Verification items for this drawing (mm, ordinates from the low corner). Round coordinates to 2 decimals unless told otherwise and drop trailing zeros. Loops run counter-clockwise (first coordinate to the right, second up) from the corner with the lowest first, then second, coordinate; pieces in that order, holes last. Notation, with made-up numbers: (14.5, 68.25) - (34.5, 68.25) arc R8 cw to (34.5, 81.25) - close; hole circle Ø4 at (38.5, 38.5). An arc over 180 degrees is marked (long way). Answer in a Markdown table with one row per item. Add a question column.
(1) Gauge pin test, flat ends, axial feed: pin 1 (3 mm diameter, centred on x = 25.5, z = 126, fed in from -Y); pin 2 (4 mm diameter, centred on x = 37.5, z = 14, fed in from -Y); pin 3 (3 mm diameter, centred on x = 23, z = 125.5, fed in from +Y); pin 4 (3 mm diameter, centred on y = 8.5, z = 29, fed in from -X). Record the tip position at first contact, or that the pin passes through.
(2) Cross-section at B-B on y = 11. Enter the section's corners in (x, z).
(3) Cross-section at C-C on x = 3. Enter the section's corners in (y, z).
(4) Thickness scan on line 1 along Z through (x, y) = (7.5, 11.75); line 2 along X through (y, z) = (14, 34.5); line 3 along X through (y, z) = (9.75, 105.5). Record the ranges inside material, lowest first.
(5) Cross-section at A-A on z = 83.5. Enter the section's corners in (x, y).
(6) Cross-section at D-D on y = 16.25. Enter the section's corners in (x, z).
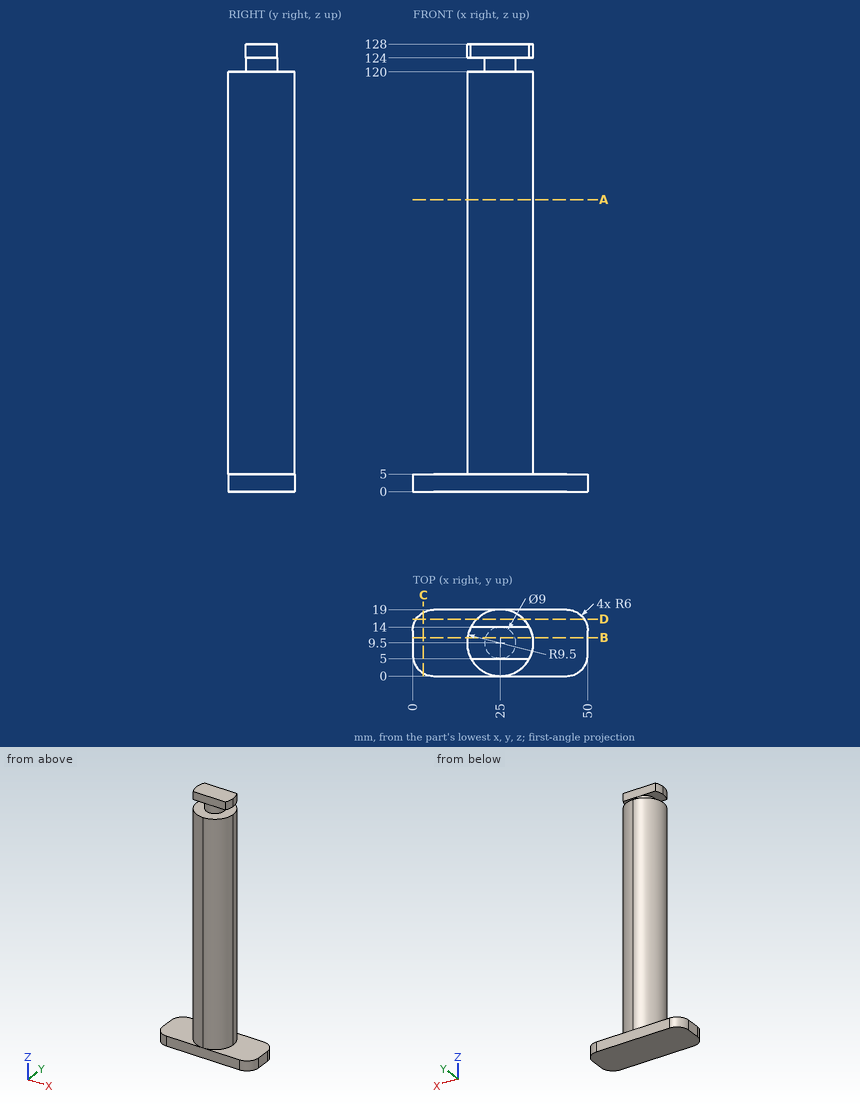
Answers:
| question | item | result |
|---|---|---|
| 1 | pin 1 | stops at y = 5 |
| 1 | pin 2 | passes through |
| 1 | pin 3 | stops at y = 14 |
| 1 | pin 4 | stops at x = 15.5 |
| 2 | outline | (0, 0) - (50, 0) - (50, 5) - (34.38, 5) - (34.38, 120) - (29.24, 120) - (29.24, 124) - (34.38, 124) - (34.38, 128) - (15.62, 128) - (15.62, 124) - (20.76, 124) - (20.76, 120) - (15.62, 120) - (15.62, 5) - (0, 5) - close |
| 3 | outline | (0.8, 0) - (18.2, 0) - (18.2, 5) - (0.8, 5) - close |
| 4 | line 1 | z = 0 to 5 |
| 4 | line 2 | x = 16.63 to 33.37 |
| 4 | line 3 | x = 15.5 to 34.5 |
| 5 | outline | circle Ø19 at (25, 9.5) |
| 6 | outline | (0.96, 0) - (49.04, 0) - (49.04, 5) - (31.68, 5) - (31.68, 120) - (18.32, 120) - (18.32, 5) - (0.96, 5) - close |
